Input: part model. Units: mm. Frame: model coordinates. Face numbers are marked on the shaded views. A direction names the side the tool comes from. Coordinates: 2 decimals unless noted, no trailing zeros. Order: outer loops, then holes, each group sorted by start corner. A loop starts at its lowest first (then second) coordinate and runs counter-clockwise, first axis right, second up. Notation, with made-up numbers: (67, 4) -> (81, 4) arc R13 ccw to (81, 29) -> close; hole circle Ø6 at (21.5, 37.25). An arc over 180 degrees is marked (long way). Use CSV: the item, a comma, the result in double quotes. Start each with the question number.
```python
from build123d import *

# Parameters (mm, degrees)
F0_R          = 10.95
F1_DEPTH      = 27
F1_DEPTH_BACK = 27
F2_R          = 8.95
F3_DEPTH      = 12
F4_SIZE       = 1
F5_R          = 8.95
F6_DEPTH      = 12
F7_SIZE       = 1


with BuildPart() as f1:
    # F0 (on Right) → F1 (new body, two sides)
    with BuildSketch(Plane.YZ) as f1_sk:
        Circle(F0_R)
    extrude(amount=F1_DEPTH)
    extrude(f1_sk.sketch, amount=-F1_DEPTH_BACK)

    # F2 (on face) → F3 (join)
    with BuildSketch(Plane.YZ.offset(27)):
        Circle(F2_R)
    extrude(amount=F3_DEPTH)

    # F4
    f4_edges = [f1.edges().sort_by_distance(p)[0] for p in [
        (39, -8.95, 0),
    ]]
    chamfer(f4_edges, length=F4_SIZE)

    # F5 (on face) → F6 (join)
    with BuildSketch(Plane(origin=(-27, 0, 0), x_dir=(0, -1, 0), z_dir=(-1, 0, 0))):
        Circle(F5_R)
    extrude(amount=F6_DEPTH)

    # F7
    f7_edges = [f1.edges().sort_by_distance(p)[0] for p in [
        (-39, 8.95, 0),
    ]]
    chamfer(f7_edges, length=F7_SIZE)


solid = f1.part
```
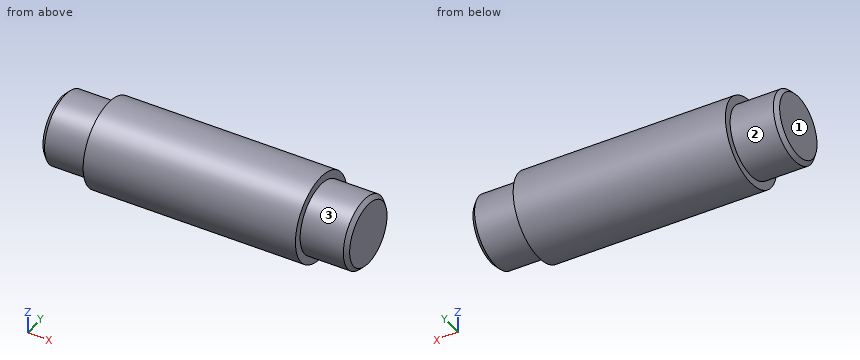
1. Access query for the marked faces 1, 2 and 3. Directions: +Z, -Z, +X, -X, +Y, -Y. A direction counts if a zero-diameter tool reaches every point of the face in a straight line with its end or side. Return the directions, or none.
2. Material intervals for line 1 along X through (y, z) = (6, 8.5); line 2 along Z through (x, y) = (30.5, -0.5); line 3 along Z through (x, y) = (20.5, 8), sorted ascending.
3. Contact query for flat-ended pins moving along their axis: P1, Ø8, axis at x = 23, y = -3.5, coming from the -Z side; P2, Ø3, axis at x = -29, y = 7.5, coming from the +Z side; P3, Ø5, axis at x = 10.5, z = 7.5, coming from the -Y side; P4, Ø1.5, axis at x = -21, z = -6, coming from the +Y side. Output: stop coordinate, or through.
4. Section A-A on y = 0. Return loops of the section in (x, z).
5. Section C-C on x = -32. Return loops of the section in (y, z), then the cut area to 3 significant figures.
6. Section D-D on x = 5. Return loops of the section in (y, z).
Values follow:
1,face 1,"+Z, -Z, -X, +Y, -Y"
1,face 2,"-X"
1,face 3,"+X"
2,line 1,"x = -27 to 27"
2,line 2,"z = -8.94 to 8.94"
2,line 3,"z = -7.48 to 7.48"
3,P1,"stops at z = -10.95"
3,P2,"stops at z = 6.64"
3,P3,"stops at y = -9.74"
3,P4,"stops at y = 9.61"
4,outline,"(-39, -7.95) -> (-38, -8.95) -> (-27, -8.95) -> (-27, -10.95) -> (27, -10.95) -> (27, -8.95) -> (38, -8.95) -> (39, -7.95) -> (39, 7.95) -> (38, 8.95) -> (27, 8.95) -> (27, 10.95) -> (-27, 10.95) -> (-27, 8.95) -> (-38, 8.95) -> (-39, 7.95) -> close"
5,outline,"circle Ø17.9 at (0, 0)"
5,area,"252 mm2"
6,outline,"circle Ø21.9 at (0, 0)"
